from build123d import *

# Parameters (mm, degrees)
F1_DEPTH = 30
F2_R     = 4.4
F3_R     = 4.4
F4_DEPTH = 25


# Not quite as in the source:
# - a feature names something its author has since deleted; it is built from what else it names


with BuildPart() as f1:
    # F0 (on Front) → F1 (new body)
    with BuildSketch(Plane.XZ):
        Polygon((90, -1), (90, 1), (70, 1), (70, 69), (-70, 69), (-70, 1), (-90, 1), (-90, -1), (-68, -1), (-68, 67), (68, 67), (68, -1), align=None)
    extrude(amount=F1_DEPTH)

    # F2 (on face) + F3 (on face) → F4 (cut)
    with BuildSketch(Plane.XY.offset(1)):
        with Locations((-80, -15)):
            Circle(F2_R)
        with Locations((80, -15)):
            Circle(F2_R)
    with BuildSketch(Plane.XY.offset(69)):
        with Locations((-37.5, -15)):
            Circle(F3_R)
        with Locations((37.5, -15)):
            Circle(F3_R)
    extrude(amount=-F4_DEPTH, mode=Mode.SUBTRACT)


solid = f1.part
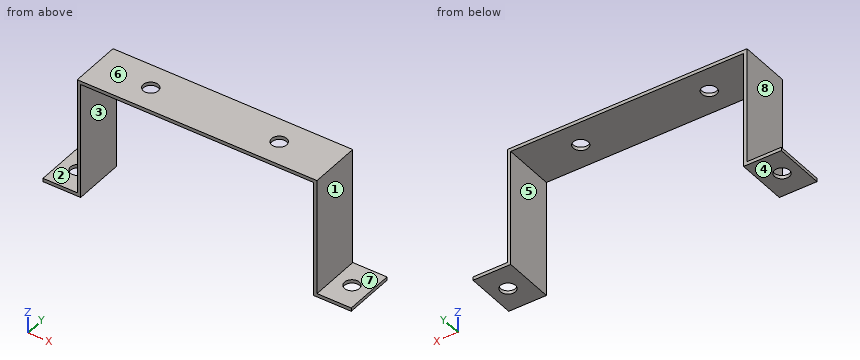
The listing builds one solid part. Answer for the finished solid, in the listing's coordinates (mm). Face numbers are marked on the shaded views. A direction names the side the tool comes from. Round coordinates to 2 decimals unless told otherwise and drop trailing zeros. Order: outer loops, then holes, each group sorted by start corner. A loop starts at its lowest first (then second) coordinate and runs counter-clockwise, first axis right, second up. Notation, with made-up numbers: M 5,42.25 L 63,42.25 A16 ccw 63,59.25 Z; hole C 2.5,70.5 d5. An arc over 180 degrees is marked long. Answer in a Markdown table with one row per item. Add a question column.
1) The part is cut by section C-C on y = -15. Determine the outline of the cut face in (x, z).
2) Determine the mould class of the marked faces 1, 2 and 3 for opening direction X: pulls with the +X half, pulls with the -X half, needs draft (parallel to the pull), parting line crosses it, or undercut.
3) Flat-ended cylindrical pins translate along their axes: pin 1 Ø15 at (x, y) = (-19.5, -10) entering from -Z; pin 2 Ø6 at (y, z) = (-26.5, 29.5) entering from -X; pin 3 Ø15 at (y, z) = (-18, 50.5) entering from +X. Find the tip coordinate at first contact, or state that the pin passes through.
4) Consider line 1 along X through (y, z) = (-20.75, 47.5); line 2 along Y through (x, z) = (-37.5, 68.5); line 3 along Z through (x, y) = (-12.5, -8). Determine where each line is inside the solid, lowest interval first. Write a range as from..to.
5) The part is cut by section D-D on x = -63. Determine the outline of the cut face in (y, z), plus the area to 3 significant figures.
6) The part is cut by section A-A on z = 60. Determine the outline of the cut face in (x, y), plus the area to 3 significant figures.
7) Which of the six approach directions +Z, -Z, +X, -X, +Y, -Y give full straight-line access (tool end or side, diameter ignored) to the marked faces 4, 5, 6, 7 and 8?
8) The part is cut by section B-B on x = 80. Determine the outline of the cut face in (y, z).
Findings below:
| question | item | result |
|---|---|---|
| 1 | outline | M -90,-1 L -84.4,-1 L -84.4,1 L -90,1 Z; M -75.6,-1 L -68,-1 L -68,67 L -41.9,67 L -41.9,69 L -70,69 L -70,1 L -75.6,1 Z; M -33.1,67 L 33.1,67 L 33.1,69 L -33.1,69 Z; M 41.9,67 L 68,67 L 68,-1 L 75.6,-1 L 75.6,1 L 70,1 L 70,69 L 41.9,69 Z; M 84.4,-1 L 90,-1 L 90,1 L 84.4,1 Z |
| 2 | face 1 | pulls with the +X half |
| 2 | face 2 | needs draft |
| 2 | face 3 | undercut |
| 3 | pin 1 | stops at z = 67 |
| 3 | pin 2 | stops at x = -70 |
| 3 | pin 3 | stops at x = 70 |
| 4 | line 1 | x = -70..-68, 68..70 |
| 4 | line 2 | y = -30..-19.4, -10.6..0 |
| 4 | line 3 | z = 67..69 |
| 5 | outline | M -30,67 L 0,67 L 0,69 L -30,69 Z |
| 5 | area | 60.0 mm² |
| 6 | outline | M -70,-30 L -68,-30 L -68,0 L -70,0 Z; M 68,-30 L 70,-30 L 70,0 L 68,0 Z |
| 6 | area | 120 mm² |
| 7 | face 4 | -Z, +X, -X, +Y, -Y |
| 7 | face 5 | -Z, +Y, -Y |
| 7 | face 6 | +Z, +X, -X, +Y, -Y |
| 7 | face 7 | +Z, +X, +Y, -Y |
| 7 | face 8 | +Z, -X, +Y, -Y |
| 8 | outline | M -30,-1 L -19.4,-1 L -19.4,1 L -30,1 Z; M -10.6,-1 L 0,-1 L 0,1 L -10.6,1 Z |
